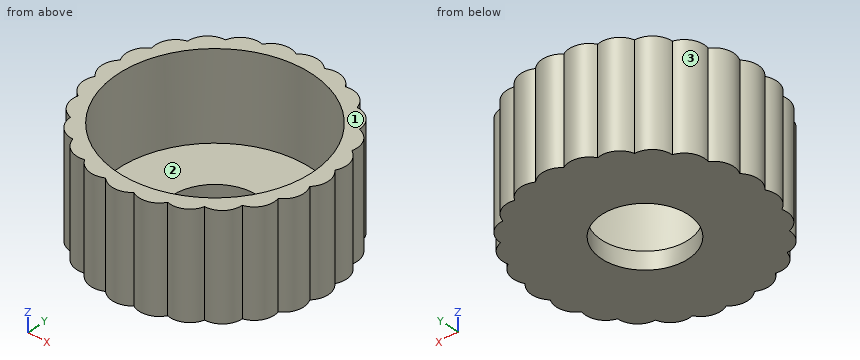
```python
from build123d import *
from build123d.topology import SkipClean

# Parameters (mm, degrees)
SKETCH1_R           = 18.75
SKETCH1_R_2         = 16.75
BOSS_EXTRUDE1_DEPTH = 15
BOSS_EXTRUDE2_START = 3
SKETCH3_R           = 18.75
SKETCH3_R_2         = 7.5
BOSS_EXTRUDE2_DEPTH = 3
BOSS_EXTRUDE3_DEPTH = 18
CIRPATTERN1_COUNT   = 24


with BuildPart() as part:
    # Sketch1 → Boss-Extrude1 (new body)
    with BuildSketch(Plane.XY):
        Circle(SKETCH1_R)
        Circle(SKETCH1_R_2, mode=Mode.SUBTRACT)
    extrude(amount=BOSS_EXTRUDE1_DEPTH)

    # Sketch3 → Boss-Extrude2 (add)
    with BuildSketch(Plane(origin=(0, 0, 0), x_dir=(-1, 0, 0), z_dir=(0, 0, -1)).offset(BOSS_EXTRUDE2_START)):
        Circle(SKETCH3_R)
        Circle(SKETCH3_R_2, mode=Mode.SUBTRACT)
    extrude(amount=-BOSS_EXTRUDE2_DEPTH)

    # Sketch4 → Boss-Extrude3 (add)
    with SkipClean():  # the faces are left unmerged after this step: merging them gives an invalid solid
        with BuildSketch(Plane(origin=(0, 0, -3), x_dir=(-1, 0, 0), z_dir=(0, 0, -1))):
            with BuildLine():
                ThreePointArc((-2.447366104, 18.589591151), (0, 19.603323383), (2.447366104, 18.589591151))
                ThreePointArc((2.447366104, 18.589591151), (0, 18.75), (-2.447366104, 18.589591151))
            make_face()
        boss_extrude3 = extrude(amount=-BOSS_EXTRUDE3_DEPTH)

    # CirPattern1: Boss-Extrude3 ×24 about axis
    with SkipClean():  # the faces are left unmerged after this step: merging them gives an invalid solid
        cirpattern1_axis = Axis((0, 0, 0), (0, 0, 1))
        for i in range(1, CIRPATTERN1_COUNT):
            add(boss_extrude3.rotate(cirpattern1_axis, i * 360 / CIRPATTERN1_COUNT))


solid = part.part
```
CAD build for the part. Positions are in the model's coordinates, mm. Face numbers are marked on the shaded views. Round coordinates to 2 decimals unless told otherwise and drop trailing zeros. Write each loop counter-clockwise with the first axis right and the second up, starting at its lowest first coordinate (ties: lowest second). Pieces come first, ordered by that corner, then holes. Notation, with made-up numbers: (52, 66.5) - (99, 66.5) arc R15 ccw to (99, 73.5) - close; hole circle Ø6 at (-22, 42.25). An arc over 180 degrees is marked (long way). Write item = value, one per line. Start each with the question number.
Q1. Band-saw the part on C-C (z = -1.25). Give the cut face in (x, y).
Q2. Mould opens along X. For the marked faces 1, 2 and 3 say: pulls with the +X half, pulls with the -X half, needs draft (parallel to the pull), parting line crosses it, or undercut.
Q3. Band-saw the part on D-D (z = 5.5). Give the cut face in (x, y), then the cut area to 3 significant figures.
Q4. Band-saw the part on A-A (x = 0). Give the cut face in (y, z), then the cut area to 3 significant figures.
Q5. Probe L1, parallel to Y at x = 0, z = 5.5; L2, parallel to Y at x = 0, z = -0.8; L3, parallel to Z at x = -13.5, y = -8. List the from-to ranges inside material, lowest first. Write a range as from..to.
Q6. Drop flat-ended pins along their axis: pin 1 (2 mm diameter, centred on y = 4.5, z = 1, fed in from -X); pin 2 (4 mm diameter, centred on y = 12.5, z = 13, fed in from -X); pin 3 (4 mm diameter, centred on y = 9.5, z = 1.5, fed in from +X); pin 4 (9 mm diameter, centred on x = 0, y = 0, fed in from -Z). Give the stop position or say it passes through.
Answers below:
q1.outline = (-18.59, -2.45) arc R3.46 ccw to (-17.32, -7.18) arc R3.46 ccw to (-14.88, -11.41) arc R3.46 ccw to (-11.41, -14.88) arc R3.46 ccw to (-7.18, -17.32) arc R3.46 ccw to (-2.45, -18.59) arc R3.46 ccw to (2.45, -18.59) arc R3.46 ccw to (7.18, -17.32) arc R3.46 ccw to (11.41, -14.88) arc R3.46 ccw to (14.88, -11.41) arc R3.46 ccw to (17.32, -7.18) arc R3.46 ccw to (18.59, -2.45) arc R3.46 ccw to (18.59, 2.45) arc R3.46 ccw to (17.32, 7.18) arc R3.46 ccw to (14.88, 11.41) arc R3.46 ccw to (11.41, 14.88) arc R3.46 ccw to (7.18, 17.32) arc R3.46 ccw to (2.45, 18.59) arc R3.46 ccw to (-2.45, 18.59) arc R3.46 ccw to (-7.18, 17.32) arc R3.46 ccw to (-11.41, 14.88) arc R3.46 ccw to (-14.88, 11.41) arc R3.46 ccw to (-17.32, 7.18) arc R3.46 ccw to (-18.59, 2.45) arc R3.46 ccw to start; hole circle Ø15 at (0, 0)
q2.face_1 = needs draft
q2.face_2 = undercut
q2.face_3 = pulls with the -X half
q3.outline = (-18.59, -2.45) arc R3.46 ccw to (-17.32, -7.18) arc R3.46 ccw to (-14.88, -11.41) arc R3.46 ccw to (-11.41, -14.88) arc R3.46 ccw to (-7.18, -17.32) arc R3.46 ccw to (-2.45, -18.59) arc R3.46 ccw to (2.45, -18.59) arc R3.46 ccw to (7.18, -17.32) arc R3.46 ccw to (11.41, -14.88) arc R3.46 ccw to (14.88, -11.41) arc R3.46 ccw to (17.32, -7.18) arc R3.46 ccw to (18.59, -2.45) arc R3.46 ccw to (18.59, 2.45) arc R3.46 ccw to (17.32, 7.18) arc R3.46 ccw to (14.88, 11.41) arc R3.46 ccw to (11.41, 14.88) arc R3.46 ccw to (7.18, 17.32) arc R3.46 ccw to (2.45, 18.59) arc R3.46 ccw to (-2.45, 18.59) arc R3.46 ccw to (-7.18, 17.32) arc R3.46 ccw to (-11.41, 14.88) arc R3.46 ccw to (-14.88, 11.41) arc R3.46 ccw to (-17.32, 7.18) arc R3.46 ccw to (-18.59, 2.45) arc R3.46 ccw to start; hole circle Ø33.5 at (0, 0)
q3.area = 293 mm2
q4.outline = (-19.6, -3) - (-7.5, -3) - (-7.5, 0) - (-16.75, 0) - (-16.75, 15) - (-19.6, 15) - close; (7.5, -3) - (19.6, -3) - (19.6, 15) - (16.75, 15) - (16.75, 0) - (7.5, 0) - close
q4.area = 158 mm2
q5.L1 = -19.6..-16.75, 16.75..19.6
q5.L2 = -19.6..-7.5, 7.5..19.6
q5.L3 = -3..0
q6.pin_1 = -19.05
q6.pin_2 = -16.45
q6.pin_3 = 17.44
q6.pin_4 = through
